Geometry check sheet. Reference: the model listing, model coordinates, mm. Face numbers are marked on the shaded views. Round coordinates to 2 decimals unless told otherwise and drop trailing zeros. Write each loop counter-clockwise with the first axis right and the second up, starting at its lowest first coordinate (ties: lowest second). Pieces come first, ordered by that corner, then holes. Notation, with made-up numbers: (-24.75, -21.5) - (-10.75, -21.5) arc R21 ccw to (-10.75, 2.5) - close; hole circle Ø7 at (-11.75, -9). An arc over 180 degrees is marked (long way). One line per question, with ' | ' between items. Start each with the question number.
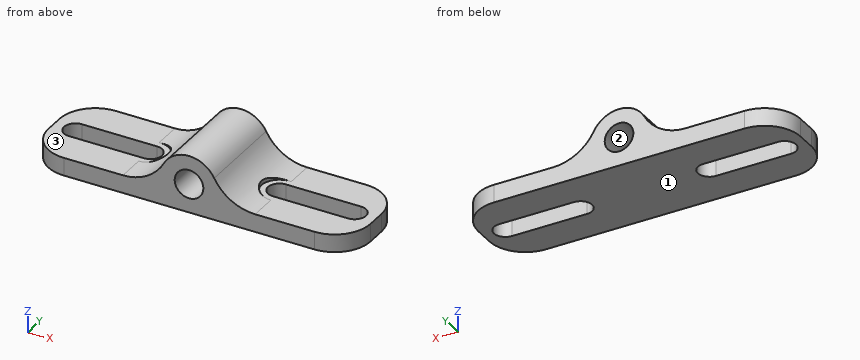
from build123d import *

# Parameters (mm, degrees)
SKETCH1_R               = 4
BOSS_EXTRUDE1_DEPTH     = 25.4
FILLET1_R               = 13
CUT_EXTRUDE1_DEPTH      = 12
CUT_EXTRUDE1_DEPTH_BACK = 6
SKETCH3_R               = 5
CUT_EXTRUDE2_DEPTH      = 25.4
FILLET2_R               = 10


with BuildPart() as part:
    # Sketch1 → Boss-Extrude1 (new body)
    with BuildSketch(Plane(origin=(0, 0, 0), x_dir=(1, 0, 0), z_dir=(0, 1, 0))):
        with BuildLine():
            Line((-45, 0), (45, 0))
            Line((45, 0), (45, -5))
            Line((45, -5), (7.416198487, -5))
            ThreePointArc((7.416198487, -5), (0, -16), (-7.416198487, -5))
            Line((-7.416198487, -5), (-45, -5))
            Line((-45, -5), (-45, 0))
        make_face()
        with Locations((0, -8)):
            Circle(SKETCH1_R, mode=Mode.SUBTRACT)
    extrude(amount=BOSS_EXTRUDE1_DEPTH)

    # Fillet1
    fillet1_edges = [part.edges().sort_by_distance(p)[0] for p in [
        (7.416198487, 12.7, 5),
        (-7.416198487, 12.7, 5),
    ]]
    fillet(fillet1_edges, radius=FILLET1_R)

    # Sketch2 → Cut-Extrude1 (cut, two sides)
    with BuildSketch(Plane.XY.offset(5)) as cut_extrude1_sk:
        with BuildLine():
            Line((-39, 15.9), (-18, 15.9))
            ThreePointArc((-18, 15.9), (-14.8, 12.7), (-18, 9.5))
            Line((-18, 9.5), (-39, 9.5))
            ThreePointArc((-39, 9.5), (-42.2, 12.7), (-39, 15.9))
        make_face()
        with BuildLine():
            Line((39, 9.5), (18, 9.5))
            ThreePointArc((18, 9.5), (14.8, 12.7), (18, 15.9))
            Line((18, 15.9), (39, 15.9))
            ThreePointArc((39, 15.9), (42.2, 12.7), (39, 9.5))
        make_face()
    extrude(amount=CUT_EXTRUDE1_DEPTH, mode=Mode.SUBTRACT)
    extrude(cut_extrude1_sk.sketch, amount=-CUT_EXTRUDE1_DEPTH_BACK, mode=Mode.SUBTRACT)

    # Sketch3 → Cut-Extrude2 (cut)
    with BuildSketch(Plane.XY.offset(5)):
        with Locations((-18, 12.7)):
            Circle(SKETCH3_R)
        with Locations((18, 12.7)):
            Circle(SKETCH3_R)
    extrude(amount=CUT_EXTRUDE2_DEPTH, mode=Mode.SUBTRACT)

    # Fillet2
    fillet2_edges = [part.edges().sort_by_distance(p)[0] for p in [
        (-45, 25.4, 2.5),
        (45, 25.4, 2.5),
        (-45, 0, 2.5),
        (45, 0, 2.5),
    ]]
    fillet(fillet2_edges, radius=FILLET2_R)


solid = part.part
Q1. Section check B-B, the plane z = 3. Record the cut outline in (x, y).
Q2. Section check C-C, the plane x = 32.5. Record the cut outline in (y, z).
Q3. Section check D-D, the plane z = 8. Record the cut outline in (x, y), then the cut area to 3 significant figures.
Q4. Go/stop test with flat-tipped pins: P1, Ø4, axis at x = 20.5, y = 18.5, coming from the +Z side; P2, Ø13, axis at x = 18, y = 12.7, coming from the +Z side; P3, Ø4, axis at y = 3, z = 5.5, coming from the -X side. Record where each tip stops, or that it passes through.
Q5. Draft check along Z on the marked faces 1, 2 and 3. Enter one of: pulls with the +Z half, pulls with the -Z half, needs draft (parallel to the pull), parting line crosses it, or undercut.
Q6. Thickness scan on line 1 (Y direction, x = -24, z = 4); line 2 (Z direction, x = 0, y = 19.5); line 3 (X direction, y = 12.7, z = 5.9). Record the ranges inside material, lowest first.
Q7. Section check A-A, the plane y = 12.7. Record the cut outline in (x, z).
Result sheet:
1) outline: (-45, 10) arc R10 ccw to (-35, 0) - (35, 0) arc R10 ccw to (45, 10) - (45, 15.4) arc R10 ccw to (35, 25.4) - (-35, 25.4) arc R10 ccw to (-45, 15.4) - close; hole (-39, 9.5) - (-18, 9.5) arc R3.2 ccw to (-18, 15.9) - (-39, 15.9) arc R3.2 ccw to start; hole (18, 9.5) - (39, 9.5) arc R3.2 ccw to (39, 15.9) - (18, 15.9) arc R3.2 ccw to start
2) outline: (0, 0) - (9.5, 0) - (9.5, 5) - (0, 5) - close; (15.9, 0) - (25.4, 0) - (25.4, 5) - (15.9, 5) - close
3) outline: (-10.16, 0) - (-4, 0) - (-4, 25.4) - (-10.16, 25.4) - close; (4, 0) - (10.16, 0) - (10.16, 25.4) - (4, 25.4) - close | area: 313 mm²
4) P1: z = 5 | P2: z = 7.02 | P3: x = -43.62
5) face 1: pulls with the -Z half | face 2: undercut | face 3: pulls with the +Z half
6) line 1: 0 to 9.5, 15.9 to 25.4 | line 2: 0 to 4, 12 to 16 | line 3: -13 to -3.4, 3.4 to 13
7) outline: (-45, 0) - (-42.2, 0) - (-42.2, 5) - (-45, 5) - close; (-14.8, 0) - (14.8, 0) - (14.8, 5) - (13, 5) - (13, 6.21) arc R13 cw to (7.03, 11.81) arc R8 ccw to (-7.03, 11.81) arc R13 cw to (-13, 6.21) - (-13, 5) - (-14.8, 5) - close; (42.2, 0) - (45, 0) - (45, 5) - (42.2, 5) - close; hole circle Ø8 at (0, 8)
